Input: part model. Units: mm. Frame: model coordinates. Face numbers are marked on the shaded views. A direction names the side the tool comes from. Coordinates: 2 decimals unless noted, no trailing zeros. Loops run counter-clockwise (first coordinate to the right, second up) from the corner with the lowest first, then second, coordinate; pieces in that order, holes last.
(1) Section C-C, the plane y = 38.75. Return loops of the section in (x, z), then the cut area to 3 significant figures.
(2) Section D-D, the plane y = 46.5. Return loops of the section in (x, z), then the cut area to 3 significant figures.
(3) Section B-B, the plane x = -38.5. Return loops of the section in (y, z).
(4) Mould query, pull axis Z, two halves, no side actions, for the marked faces 1, 2 and 3. Classes: released by +Z, released by -Z, zero draft, split by the parting line, or undercut.
(5) Contact query for flat-ended pins moving along their axis: P1, Ø0.6, axis at x = -33.5, y = 50, coming from the +Z side; P2, Ø2, axis at x = -35.5, y = 27, coming from the -Z side; P3, Ø5.5, axis at x = -33, y = 44, coming from the -Z side; P4, Ø1, axis at x = -34, z = -2, coming from the -Y side. Output: stop coordinate, or through.
(6) Section A-A, the plane z = 14. Return loops of the section in (x, y).
(7) Line query: L1, parallel to Z at x = -32.75, y = 40.75; L2, parallel to Z at x = -32.25, y = 34; L3, parallel to Z at x = -35.25, y = 33.75. Output: solid intervals per line, ascending.
(8) Set-up query: the marked faces 4, 5, 6, 7 and 8. Return all of +Z, -Z, +X, -X, +Y, -Y with unobstructed straight access to the full face (end or side cutting, diameter ignored); none if empty.
```python
from build123d import *

# Parameters (mm, degrees)
SKETCH052_W             = 10
SKETCH052_H             = 20
PAD024_DEPTH            = 5
SKETCH049_W             = 10
SKETCH049_H             = 10
PAD023_DEPTH            = 6
SKETCH050_W             = 24
SKETCH050_H             = 22
PAD025_DEPTH            = 5
SKETCH048_W             = 16
SKETCH048_H             = 18
POCKET019_DEPTH         = 6
SKETCH051_R             = 3.7
POCKET018_DEPTH         = 10
SKETCH053_W             = 10
SKETCH053_H             = 5
PAD026_DEPTH            = 2
SKETCH064_R             = 9
POCKET024_DEPTH         = 5
BODY010_PLACEMENT_ANGLE = 180


with BuildPart() as part:
    # Sketch052 → Pad024 (new body)
    with BuildSketch(Plane.XY):
        with Locations((0, -2.5)):
            Rectangle(SKETCH052_W, SKETCH052_H)
    extrude(amount=PAD024_DEPTH)

    # Sketch049 → Pad023 (join)
    with BuildSketch(Plane.XY):
        Rectangle(SKETCH049_W, SKETCH049_H)
    extrude(amount=PAD023_DEPTH)

    # Sketch050 → Pad025 (join, symmetric)
    with BuildSketch(Plane.YZ):
        with Locations((0, 16)):
            Rectangle(SKETCH050_W, SKETCH050_H)
    extrude(amount=PAD025_DEPTH, both=True)

    # Sketch048 → Pocket019 (cut)
    with BuildSketch(Plane.YZ):
        with Locations((-8, 15)):
            Rectangle(SKETCH048_W, SKETCH048_H)
    extrude(amount=-POCKET019_DEPTH, mode=Mode.SUBTRACT)

    # Sketch051 → Pocket018 (cut, symmetric)
    with BuildSketch(Plane.YZ):
        with Locations((0, 15)):
            Circle(SKETCH051_R)
    extrude(amount=POCKET018_DEPTH, both=True, mode=Mode.SUBTRACT)

    # Sketch053 → Pad026 (join)
    with BuildSketch(Plane.XY):
        with Locations((0, -2.5)):
            Rectangle(SKETCH053_W, SKETCH053_H)
    extrude(amount=-PAD026_DEPTH)

    # Sketch064 → Pocket024 (cut)
    with BuildSketch(Plane.YZ):
        with Locations((0, 15)):
            Circle(SKETCH064_R)
    extrude(amount=-POCKET024_DEPTH, mode=Mode.SUBTRACT)


with BuildPart() as part_1:
    # Body010 placement: moved
    add(part.part.moved(Location((-35, 37.5, -1))).rotate(Axis((-35, 37.5, -1), (0, 0, 1)), BODY010_PLACEMENT_ANGLE))


solid = part_1.part
```
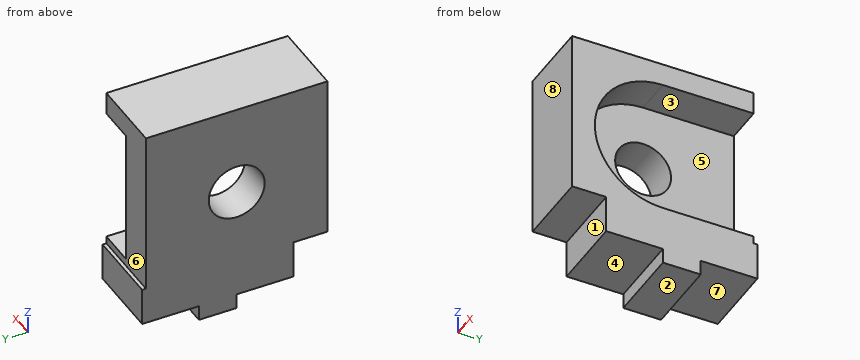
Report:
1. outline: (-40, -3) - (-30, -3) - (-30, 5) - (-35, 5) - (-35, 10.52) - (-40, 10.52) - close; (-40, 17.48) - (-35, 17.48) - (-35, 23) - (-30, 23) - (-30, 26) - (-40, 26) - close
1. area: 165 mm2
2. outline: (-40, -1) - (-30, -1) - (-30, 5) - (-35, 5) - (-35, 23) - (-30, 23) - (-30, 26) - (-40, 26) - close
2. area: 180 mm2
3. outline: (25.5, 4) - (30, 4) - (30, -1) - (37.5, -1) - (37.5, -3) - (42.5, -3) - (42.5, -1) - (50, -1) - (50, 4) - (49.5, 4) - (49.5, 26) - (25.5, 26) - close; hole circle Ø7.4 at (37.5, 14)
4. face 1: zero draft
4. face 2: released by -Z
4. face 3: undercut
5. P1: stops at z = 4
5. P2: stops at z = 4
5. P3: stops at z = -3
5. P4: stops at y = 37.5
6. outline: (-40, 25.5) - (-30, 25.5) - (-30, 28.5) - (-35, 28.5) - (-35, 33.8) - (-40, 33.8) - close; (-40, 41.2) - (-35, 41.2) - (-35, 49.5) - (-40, 49.5) - close
7. L1: z = -3 to 5, 23 to 26
7. L2: z = -1 to 5.71, 22.29 to 26
7. L3: z = -1 to 26
8. face 4: -Z, +X, -X, -Y
8. face 5: +X, +Y
8. face 6: +Z, +X, -X, +Y
8. face 7: -Z, +X, -X, +Y
8. face 8: +Z, -Z, +X, -X, -Y
